Read the model definition and answer for the solid it produces. Units are mm, in the model's axes. A direction names the side the tool comes from. Coordinates: 2 decimals unless noted, no trailing zeros. Loops run counter-clockwise (first coordinate to the right, second up) from the corner with the lowest first, then second, coordinate; pieces in that order, holes last. Notation, with made-up numbers: (29, -22) -> (87, -22) arc R31 ccw to (87, 6) -> close; hole circle Ø5 at (82, 77). An arc over 180 degrees is marked (long way). Answer as a JSON object with one key per item and string values. Group by question number.
1) Consider probe 1 along X at (y, z) = (29.5, 15); probe 2 along Z at (x, y) = (44, 29); probe 3 along Z at (x, y) = (-3, 29). Determine where each line is inside the solid, lowest interval first. Write a range as [from, to].
2) Which of the six approach directions +Z, -Z, +X, -X, +Y, -Y give full straight-line access (tool end or side, diameter ignored) to faces 4 (the face through (-3, 31, 10)), 5 (the face through (-3, 28, 10)), 6 (the face through (40.3, 33, 10)), 7 (the face through (7.56, 39.94, 9.46)), 8 (the face through (44, 28, 10))?
3) Section C-C, the plane z = 8.5 is taken. Give the vertices of the cut face in (x, y).
4) Determine the mould class of faces 1 (the face through (0, 14, 10)), 2 (the face through (40.3, 14, 10)), 3 (the face through (-5.067, 29.479, 3.413)) for opening direction X: released by +X, released by -X, zero draft, split by the parting line, or undercut.
5) Section A-A, the plane x = 44.15 is taken. Give the vertices of the cut face in (y, z).
6) Section D-D, the plane x = 10 is taken. Give the vertices of the cut face in (y, z).
7) Section B-B, the plane z = 15 is taken. Give the vertices of the cut face in (x, y), plus the area to 3 significant figures.
8) Flat-ended cylindrical pins translate along their axes: P1, Ø5, axis at y = 9.5, z = 13.5, coming from the +X side; P2, Ø10, axis at x = 24, z = 14.5, coming from the +Y side; P3, Ø1, axis at y = 35, z = 13, coming from the -X side. Find the tip coordinate at first contact, or state that the pin passes through.
from build123d import *

# Parameters (mm, degrees)
SKETCH1_W           = 40.3
SKETCH1_H           = 20
BOSS_EXTRUDE1_DEPTH = 28
SKETCH2_R           = 2
BOSS_EXTRUDE2_DEPTH = 3
SKETCH3_W           = 40.3
SKETCH3_H           = 20
BOSS_EXTRUDE3_DEPTH = 8
SKETCH4_R           = 2.5
BOSS_EXTRUDE4_DEPTH = 8


with BuildPart() as part:
    # Sketch1 → Boss-Extrude1 (new body)
    with BuildSketch(Plane(origin=(0, 0, 0), x_dir=(1, 0, 0), z_dir=(0, 1, 0))):
        with Locations((20.15, -10)):
            Rectangle(SKETCH1_W, SKETCH1_H)
    extrude(amount=BOSS_EXTRUDE1_DEPTH)

    # Sketch2 → Boss-Extrude2 (add)
    with BuildSketch(Plane(origin=(0, 28, 0), x_dir=(1, 0, 0), z_dir=(0, 1, 0))):
        Polygon((20.15, 0), (-6.85, 0), (-6.85, -20), (20.15, -20), (47.15, -20), (47.15, 0), align=None)
        with Locations(Location((-3.85, -5, 0), (0, 0, 270))):
            Circle(SKETCH2_R, mode=Mode.SUBTRACT)
        with Locations(Location((-3.85, -15, 0), (0, 0, 270))):
            Circle(SKETCH2_R, mode=Mode.SUBTRACT)
        with Locations(Location((44.15, -5, 0), (0, 0, 270))):
            Circle(SKETCH2_R, mode=Mode.SUBTRACT)
        with Locations(Location((44.15, -15, 0), (0, 0, 270))):
            Circle(SKETCH2_R, mode=Mode.SUBTRACT)
    extrude(amount=BOSS_EXTRUDE2_DEPTH)

    # Sketch3 → Boss-Extrude3 (add)
    with BuildSketch(Plane(origin=(0, 28, 0), x_dir=(1, 0, 0), z_dir=(0, 1, 0))):
        with Locations((20.15, -10)):
            Rectangle(SKETCH3_W, SKETCH3_H)
    extrude(amount=BOSS_EXTRUDE3_DEPTH)

    # Sketch4 → Boss-Extrude4 (add)
    with BuildSketch(Plane(origin=(0, 36, 0), x_dir=(1, 0, 0), z_dir=(0, 1, 0))):
        with Locations(Location((10, -10, 0), (0, 0, 270))):
            Circle(SKETCH4_R)
    extrude(amount=BOSS_EXTRUDE4_DEPTH)


solid = part.part
Determined:
{
 "1": {"probe 1": "[-6.85, -5.85], [-1.85, 42.15], [46.15, 47.15]", "probe 2": "[0, 3.01], [6.99, 13.01], [16.99, 20]", "probe 3": "[0, 3.19], [6.81, 13.19], [16.81, 20]"},
 "2": {"face 4": "+Z, -Z, -X, +Y", "face 5": "+Z, -Z, -X, -Y", "face 6": "+Z, -Z, +X, +Y", "face 7": "+Y", "face 8": "+Z, -Z, +X, -Y"},
 "3": {"outline": "(-6.85, 28) -> (0, 28) -> (0, 0) -> (40.3, 0) -> (40.3, 28) -> (47.15, 28) -> (47.15, 31) -> (40.3, 31) -> (40.3, 36) -> (12, 36) -> (12, 44) -> (8, 44) -> (8, 36) -> (0, 36) -> (0, 31) -> (-6.85, 31) -> close"},
 "4": {"face 1": "released by -X", "face 2": "released by +X", "face 3": "undercut"},
 "5": {"outline": "(28, 0) -> (31, 0) -> (31, 3) -> (28, 3) -> close; (28, 7) -> (31, 7) -> (31, 13) -> (28, 13) -> close; (28, 17) -> (31, 17) -> (31, 20) -> (28, 20) -> close"},
 "6": {"outline": "(0, 0) -> (36, 0) -> (36, 7.5) -> (44, 7.5) -> (44, 12.5) -> (36, 12.5) -> (36, 20) -> (0, 20) -> close"},
 "7": {"outline": "(-6.85, 28) -> (-5.85, 28) -> (-5.85, 31) -> (-6.85, 31) -> close; (-1.85, 28) -> (0, 28) -> (0, 0) -> (40.3, 0) -> (40.3, 28) -> (42.15, 28) -> (42.15, 31) -> (40.3, 31) -> (40.3, 36) -> (0, 36) -> (0, 31) -> (-1.85, 31) -> close; (46.15, 28) -> (47.15, 28) -> (47.15, 31) -> (46.15, 31) -> close", "area": "1,470 mm²"},
 "8": {"P1": "x = 40.3", "P2": "y = 36", "P3": "x = 0"}
}
